Model file for the job. Use its own axes, mm. A direction names the side the tool comes from. Coordinates: 2 decimals unless noted, no trailing zeros. Write each loop counter-clockwise with the first axis right and the second up, starting at its lowest first coordinate (ties: lowest second). Pieces come first, ordered by that corner, then holes.
Q1. Which spindle directions (+Z, -Z, +X, -X, +Y, -Y) get a long thin tool onto all of the face, cutting with end or side? Do faces 5 (the flat face through (31, 0, -6.3)), 6 (the flat face through (320.1, 31.25, 9.1)). Say none if no direction does.
Q2. Drill centre lines: probe 1 along X at (y, z) = (-25.5, -1); probe 2 along X at (y, z) = (-3, 0); probe 3 along Z at (x, y) = (300, 16). Where is each one in solid material? Low to high.
Q3. Band-saw the part on C-C, the plane y = 1. Write the cut outline in (x, z), plus the area to 3 significant figures.
Q4. Pull direction Z, two halves, no side cores. Call faces 1 (the flat face through (154.18, 0.18, 49.87)), 2 (the flat face through (320.1, -31.25, 9.1)), 3 (the flat face through (35, 0, 0)), 4 (the flat face through (31, 0, 6.3)): released by +Z, released by -Z, zero draft, split by the parting line, or undercut.
Q5. Pin check, flat tips, straight feed: P1, Ø6, axis at x = 301.5, y = -9.5, coming from the -Z side; P2, Ø8.5, axis at x = 33, y = -7, coming from the -Z side; P3, Ø5, axis at y = -3, z = -10, coming from the +X side; P4, Ø4, axis at y = 5.5, z = -1.5, coming from the -X side. Stop position of each tip, or through.
Q6. Band-saw the part on A-A, the plane z = 0. Write the cut outline in (x, y), plus the area to 3 significant figures.
Q7. Band-saw the part on D-D, the plane x = -7. Write the cut outline in (y, z), plus the area to 3 significant figures.
Q8. Band-saw the part on B-B, the plane y = 16. Write the cut outline in (x, z), plus the area to 3 significant figures.
from build123d import *

# Parameters (mm, degrees)
SKETCH1_R           = 21.9
BOSS_EXTRUDE1_DEPTH = 31.25
CUT_EXTRUDE1_DEPTH  = 18.75


with BuildPart() as part:
    # Sketch1 → Boss-Extrude1 (new body, symmetric)
    with BuildSketch(Plane(origin=(0, 0, 0), x_dir=(1, 0, 0), z_dir=(0, 1, 0))):
        with BuildLine():
            Line((2.34375, 56.201150664), (301.822916667, 43.712006072))
            ThreePointArc((301.822916667, 43.712006072), (343.75, 0), (301.822916667, -43.712006072))
            Line((301.822916667, -43.712006072), (2.34375, -56.201150664))
            ThreePointArc((2.34375, -56.201150664), (-56.25, 0), (2.34375, 56.201150664))
        make_face()
        with Locations((300, 0)):
            Circle(SKETCH1_R, mode=Mode.SUBTRACT)
        with BuildLine():
            Line((27.435970914, 6.3), (35, 6.3))
            Line((35, 6.3), (35, -6.3))
            Line((35, -6.3), (27.435970914, -6.3))
            ThreePointArc((27.435970914, -6.3), (-28.15, 0), (27.435970914, 6.3))
        make_face(mode=Mode.SUBTRACT)
    extrude(amount=BOSS_EXTRUDE1_DEPTH, both=True)

    # Sketch2 → Cut-Extrude1 (cut)
    with BuildSketch(Plane(origin=(0, 31.25, 0), x_dir=(1, 0, 0), z_dir=(0, 1, 0))):
        with BuildLine():
            Line((2.34375, 56.201150664), (301.822916667, 43.712006072))
            ThreePointArc((301.822916667, 43.712006072), (256.25, 0), (301.822916667, -43.712006072))
            Line((301.822916667, -43.712006072), (2.34375, -56.201150664))
            ThreePointArc((2.34375, -56.201150664), (56.25, 0), (2.34375, 56.201150664))
        make_face()
    cut_extrude1 = extrude(amount=-CUT_EXTRUDE1_DEPTH, mode=Mode.SUBTRACT)

    # Mirror1: Cut-Extrude1 across plane
    add(cut_extrude1.mirror(Plane.ZX), mode=Mode.SUBTRACT)


solid = part.part
Answer sheet:
1. face 5: +Y, -Y
1. face 6: +Z, -Z, +X, -X, +Y
2. probe 1: x = -56.24 to -28.13, 35 to 56.24, 256.26 to 278.12, 321.88 to 343.74
2. probe 2: x = -56.25 to -28.15, 35 to 278.1, 321.9 to 343.75
2. probe 3: z = -43.75 to -21.9, 21.9 to 43.75
3. outline: (2.34, -56.2) - (301.82, -43.71) arc R43.75 ccw to (301.82, 43.71) - (2.34, 56.2) arc R56.25 ccw (long way) to start; hole (27.44, -6.3) - (35, -6.3) - (35, 6.3) - (27.44, 6.3) arc R28.15 ccw (long way) to start; hole circle Ø43.8 at (300, 0)
3. area: 33,900 mm2
4. face 1: released by +Z
4. face 2: zero draft
4. face 3: undercut
4. face 4: undercut
5. P1: stops at z = -43.85
5. P2: stops at z = -55.1
5. P3: stops at x = 343.1
5. P4: stops at x = -56.25
6. outline: (-56.25, -31.25) - (-28.15, -31.25) - (-28.15, 31.25) - (-56.25, 31.25) - close; (35, -31.25) - (56.25, -31.25) - (56.25, -12.5) - (256.25, -12.5) - (256.25, -31.25) - (278.1, -31.25) - (278.1, 31.25) - (256.25, 31.25) - (256.25, 12.5) - (56.25, 12.5) - (56.25, 31.25) - (35, 31.25) - close; (321.9, -31.25) - (343.75, -31.25) - (343.75, 31.25) - (321.9, 31.25) - close
6. area: 10,800 mm2
7. outline: (-31.25, -55.81) - (31.25, -55.81) - (31.25, -27.27) - (-31.25, -27.27) - close; (-31.25, 27.27) - (31.25, 27.27) - (31.25, 55.81) - (-31.25, 55.81) - close
7. area: 3,570 mm2
8. outline: circle Ø112.5 at (0, 0); circle Ø87.5 at (300, 0); hole (27.44, -6.3) - (35, -6.3) - (35, 6.3) - (27.44, 6.3) arc R28.15 ccw (long way) to start; hole circle Ø43.8 at (300, 0)
8. area: 11,900 mm2
